Here's the drawing with two shaded views (mm, measured from the low corner). I have some questions. Round coordinates to 2 decimals unless told otherwise and drop trailing zeros. Loops run counter-clockwise (first coordinate to the right, second up) from the corner with the lowest first, then second, coordinate; pieces in that order, holes last. Notation, with made-up numbers: (61.25, -10) - (87.25, -10) arc R18 ccw to (87.25, 1) - close; hole circle Ø10 at (-4.5, 86.5). An arc over 180 degrees is marked (long way). Use one line per item in the form item = value.
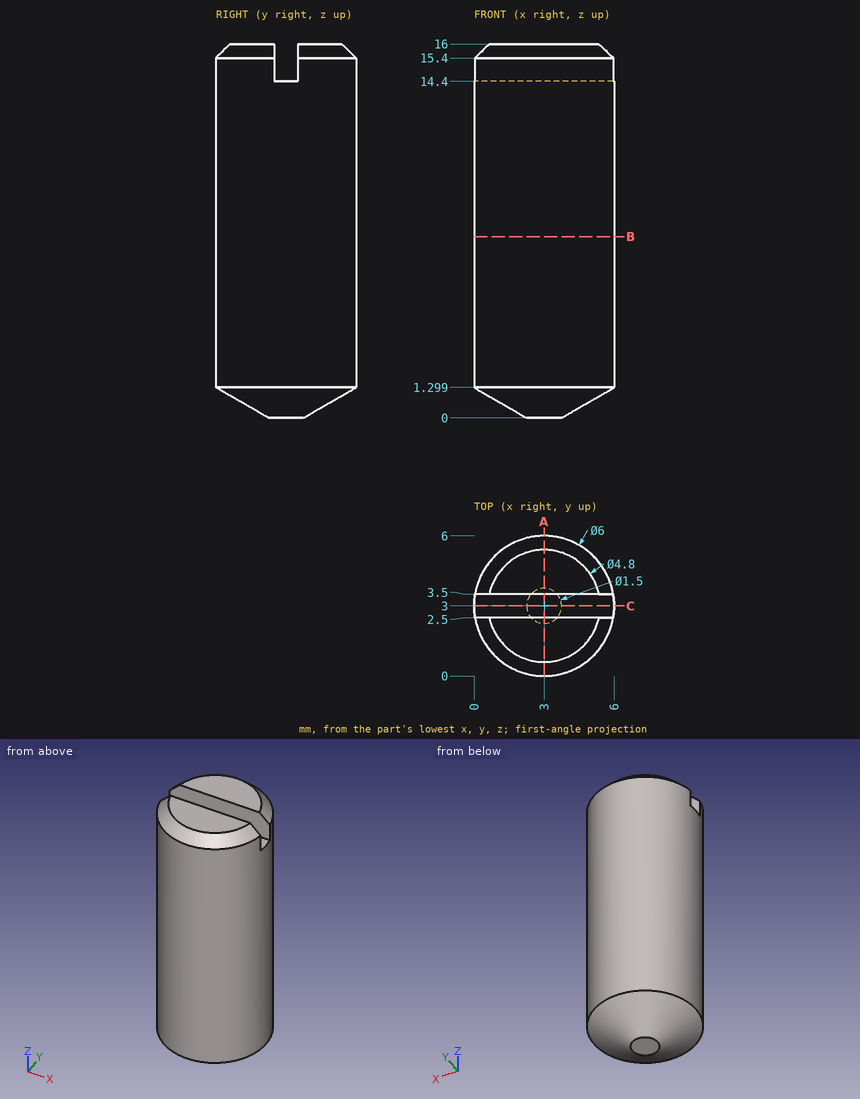
1. If we section it at A-A, the plane x = 3: Write out the boundary of the cut face in (y, z), plus the area to 3 significant figures.
Solution:
outline = (0, 1.3) - (2.25, 0) - (3.75, 0) - (6, 1.3) - (6, 15.4) - (5.4, 16) - (3.5, 16) - (3.5, 14.4) - (2.5, 14.4) - (2.5, 16) - (0.6, 16) - (0, 15.4) - close
area = 91.1 mm^2
2. If we section it at C-C, the plane y = 3: Write out the boundary of the cut face in (x, z), plus the area to 3 significant figures.
Solution:
outline = (0, 1.3) - (2.25, 0) - (3.75, 0) - (6, 1.3) - (6, 14.4) - (0, 14.4) - close
area = 83.5 mm^2
3. If we section it at B-B, the plane z = 7.75: Write out the boundary of the cut face in (x, y).
Solution:
outline = circle Ø6 at (3, 3)
4. Please list where these lines run through material, in increasing order: line 1 along X through (y, z) = (3.1, 7.25); line 2 along Y through (x, z) = (2.8, 15); line 3 along X through (y, z) = (3.55, 7.75).
Solution:
line_1 = 0 to 6
line_2 = 0.01 to 2.5, 3.5 to 5.99
line_3 = 0.05 to 5.95
5. For P1, Ø1.3, axis at x = 2.5, z = 15, coming from the +Y side; P2, Ø1.5, axis at x = 1.5, z = 14, coming from the +Y side; P3, Ø1.8, axis at x = 1.5, z = 15, coming from the -Y side; P4, Ø1.5, axis at x = 1, z = 11, coming from the +Y side, each with a flat end and sliding along its axis, tell me the tip position at first contact or that it passes through.
Solution:
P1 = 6
P2 = 5.9
P3 = 0.06
P4 = 5.73
